Geometry: final body of the model. Coordinates: model frame, mm. A direction names the side the tool comes from. Round coordinates to 2 decimals unless told otherwise and drop trailing zeros. Loops run counter-clockwise (first coordinate to the right, second up) from the corner with the lowest first, then second, coordinate; pieces in that order, holes last. Notation, with made-up numbers: (62, 23.5) - (121, 23.5) arc R27 cw to (121, 44.5) - close; hole circle Ø3 at (11.25, -34.5). An arc over 180 degrees is marked (long way). Write item = value, one per line. Start each with the question number.
Item 1: Section B-B (x = -2542.5). Return loops of the section in (y, z), plus the area to 3 significant figures.
Item 2: Section A-A (z = 334). Return loops of the section in (x, y), plus the area to 3 significant figures.
Item 3: First-contact query: pin 1 (5 mm diameter, centred on x = -2515, y = -1120.5, fed in from -Z). Flat tip, straight axial feed; report the tip coordinate or a pass-through.
Item 4: Draft query along Y for faces 1 (the flat face through (-2672, 125, 0)), 2 (the flat face through (-2672, 86.587, 301)), 3 (the flat face through (-2672, -2351.813, 301)), 4 (the flat face through (-2672, -2428.013, 338)). Return one class per face: pulls with the +Y half, pulls with the -Y half, needs draft (parallel to the pull), parting line crosses it, or undercut.
Item 5: Access query for faces 5 (the flat face through (-2672, 162.787, 338)), 6 (the flat face through (-2672, -1116, 609.6)). Directions: +Z, -Z, +X, -X, +Y, -Y. A direction counts if a zero-diameter tool reaches every point of the face in a straight line with its end or side. Return the directions, or none.
Item 6: Line query: line 1 (Y direction, x = -2581.5, z = 455); line 2 (Z direction, x = -2504, y = -1866). Output: solid intervals per line, ascending. Write a range as from..to.
Item 7: Section C-C (y = -174). Return loops of the section in (x, z), plus the area to 3 significant figures.
from build123d import *

# Parameters (mm, degrees)
F0_W     = 457.2
F0_H     = 2438.4
F1_DEPTH = 609.6
F2_T     = 76.2


with BuildPart() as f1:
    # F0 (on Top) → F1 (new body)
    with BuildSketch(Plane.XY):
        with Locations((-2668.6739219427, -1132.6131924457)):
            Rectangle(F0_W, F0_H)
    extrude(amount=F1_DEPTH)

    # F2
    f2_openings = [f1.faces().sort_by_distance(p)[0] for p in [
        (-2440.073922, -1132.613192, 304.8),
        (-2897.273922, -1132.613192, 304.8),
        (-2668.673922, -1132.613192, 0),
    ]]
    offset(amount=F2_T, openings=f2_openings, kind=Kind.INTERSECTION)


solid = f1.part
Taken from the geometry:
q1.outline = (-2428.01, 0) - (-2351.81, 0) - (-2351.81, 609.6) - (86.59, 609.6) - (86.59, 0) - (162.79, 0) - (162.79, 685.8) - (-2428.01, 685.8) - close
q1.area = 290,000 mm^2
q2.outline = (-2897.27, -2428.01) - (-2440.07, -2428.01) - (-2440.07, -2351.81) - (-2897.27, -2351.81) - close; (-2897.27, 86.59) - (-2440.07, 86.59) - (-2440.07, 162.79) - (-2897.27, 162.79) - close
q2.area = 69,700 mm^2
q3.pin_1 = 609.6
q4.face_1 = needs draft
q4.face_2 = undercut
q4.face_3 = undercut
q4.face_4 = pulls with the -Y half
q5.face_5 = +Z, -Z, +X, -X, +Y
q5.face_6 = -Z, +X, -X
q6.line_1 = -2428.01..-2351.81, 86.59..162.79
q6.line_2 = 609.6..685.8
q7.outline = (-2897.27, 609.6) - (-2440.07, 609.6) - (-2440.07, 685.8) - (-2897.27, 685.8) - close
q7.area = 34,800 mm^2
